```python
from build123d import *

# Parameters (mm, degrees)
SKETCH1_W           = 12.41763252
SKETCH1_H           = 12.769068876
SKETCH1_R           = 1.5
BOSS_EXTRUDE1_DEPTH = 13.7
SKETCH2_R           = 1.5
CUT_EXTRUDE1_DEPTH  = 23.47079699
CUT_EXTRUDE2_DEPTH  = 1.8
SKETCH5_W           = 1.8
SKETCH5_H           = 5.542562584
CUT_EXTRUDE4_DEPTH  = 3.769069
SKETCH6_W           = 1.8
SKETCH6_H           = 2.771281292
CUT_EXTRUDE5_DEPTH  = 17.740669043


with BuildPart() as part:
    # Sketch1 → Boss-Extrude1 (new body)
    # profile 1 of 2: a face of its own
    with BuildSketch(Plane.XY):
        with Locations((0.79118374, 6.384534438)):
            Rectangle(SKETCH1_W, SKETCH1_H)
        with Locations(Location((1.465537563, 5, 0), (0, 0, 180))):
            Circle(SKETCH1_R, mode=Mode.SUBTRACT)
        with Locations((1.465537563, 10)):
            Circle(SKETCH1_R, mode=Mode.SUBTRACT)
    # profile 2 of 2: a face of its own
    with BuildSketch(Plane.XY):
        with Locations((1.465537563, 10)):
            Circle(SKETCH1_R)
    extrude(amount=BOSS_EXTRUDE1_DEPTH)

    # Sketch2 → Cut-Extrude1 (cut, through all)
    with BuildSketch(Plane.ZY.offset(5.41763252)):
        with Locations((6.85, 9)):
            Circle(SKETCH2_R)
    extrude(amount=-CUT_EXTRUDE1_DEPTH, mode=Mode.SUBTRACT)

    # Sketch3 → Cut-Extrude2 (cut)
    with BuildSketch(Plane(origin=(-3.41763252, 0, 0), x_dir=(0, 0, -1), z_dir=(1, 0, 0))):
        Polygon((-5.464359354, 6.6), (-4.078718708, 9), (-5.464359354, 11.4), (-8.235640646, 11.4), (-9.621281292, 9), (-8.235640646, 6.6), align=None)
    extrude(amount=CUT_EXTRUDE2_DEPTH, mode=Mode.SUBTRACT)

    # Sketch5 → Cut-Extrude4 (cut)
    with BuildSketch(Plane(origin=(0, 12.769068876, 0), x_dir=(1, 0, 0), z_dir=(0, 1, 0))):
        with Locations((-2.51763252, -6.85)):
            Rectangle(SKETCH5_W, SKETCH5_H)
    extrude(amount=-CUT_EXTRUDE4_DEPTH, mode=Mode.SUBTRACT)

    # Sketch6 → Cut-Extrude5 (cut, through all)
    with BuildSketch(Plane(origin=(0, 6.6, 0), x_dir=(1, 0, 0), z_dir=(0, 1, 0))):
        with Locations((-2.51763252, -6.85)):
            Rectangle(SKETCH6_W, SKETCH6_H)
    extrude(amount=-CUT_EXTRUDE5_DEPTH, mode=Mode.SUBTRACT)


solid = part.part
```
Input: part model. Units: mm. Frame: model coordinates. A direction names the side the tool comes from. Coordinates: 2 decimals unless noted, no trailing zeros. Loops run counter-clockwise (first coordinate to the right, second up) from the corner with the lowest first, then second, coordinate; pieces in that order, holes last.
Q1. Section C-C, the plane y = 11.5. Return the cut outline in (x, z).
Results are:
outline: (-5.42, 0) - (7, 0) - (7, 13.7) - (-5.42, 13.7) - close; hole (-3.42, 4.08) - (-1.62, 4.08) - (-1.62, 9.62) - (-3.42, 9.62) - close
Q2. Section A-A, the plane y = 5. Return the cut outline in (x, z).
Results are:
outline: (-5.42, 0) - (-0.03, 0) - (-0.03, 13.7) - (-5.42, 13.7) - close; (2.97, 0) - (7, 0) - (7, 13.7) - (2.97, 13.7) - close; hole (-3.42, 5.46) - (-1.62, 5.46) - (-1.62, 8.24) - (-3.42, 8.24) - close
Q3. Contact query for a flat-ended pin moving along its axis: pin 1 (2.5 mm diameter, centred on x = 1.47, y = 5, fed in from -Z). Output: stop coordinate, or through.
Results are:
pin 1: passes through
Q4. Mould query, pull axis Z, two halves, no side actions, for faces 4 (the cylindrical face through (0.035, 4.549, 6.754)), 5 (the flat face through (-3, 3, 8.236)), 6 (the flat face through (0.7, 6.5, 0)). Classes: +Z half, -Z half, draft (parallel to the pull), parting line (faces both ways), or undercut.
Results are:
face 4: draft
face 5: undercut
face 6: -Z half
Q5. Section D-D, the plane x = -2.25. Return the cut outline in (y, z).
Results are:
outline: (0, 0) - (12.77, 0) - (12.77, 4.08) - (9, 4.08) - (6.6, 5.46) - (0, 5.46) - close; (0, 8.24) - (6.6, 8.24) - (9, 9.62) - (12.77, 9.62) - (12.77, 13.7) - (0, 13.7) - close
Q6. Line query: line 1 along Z through (x, y) = (-2.5, 2.75); line 2 along Y through (x, z) = (5, 6.85); line 3 along X through (y, z) = (7.5, 8). Output: solid intervals per line, ascending.
Results are:
line 1: z = 0 to 5.46, 8.24 to 13.7
line 2: y = 0 to 7.5, 10.5 to 12.77
line 3: x = -5.42 to -3.42, -1.62 to 7
Q7. Section B-B, the plane z = 6.85. Return the cut outline in (x, y).
Results are:
outline: (-5.42, 0) - (-3.42, 0) - (-3.42, 7.5) - (-5.42, 7.5) - close; (-5.42, 10.5) - (-3.42, 10.5) - (-3.42, 12.77) - (-5.42, 12.77) - close; (-1.62, 0) - (7, 0) - (7, 7.5) - (-1.62, 7.5) - close; (-1.62, 10.5) - (7, 10.5) - (7, 12.77) - (-1.62, 12.77) - close; hole circle Ø3 at (1.47, 5)
Q8. Set-up query: faces 1 (the flat face through (0.7, 6.5, 13.7)), 2 (the flat face through (-3, 11, 4.079)), 3 (the flat face through (-3, 3, 5.464)). Return all of +Z, -Z, +X, -X, +Y, -Y with unobstructed straight access to the full face (end or side cutting, diameter ignored); none if empty.
Results are:
face 1: +Z, +X, -X, +Y, -Y
face 2: +Y
face 3: +Y, -Y
